```python
from build123d import *

# Parameters (mm, degrees)
SKETCH1_W           = 35
SKETCH1_H           = 35
BOSS_EXTRUDE1_DEPTH = 1
SKETCH3_R           = 11.5
SKETCH3_R_2         = 10.25
BOSS_EXTRUDE3_DEPTH = 10
FILLET1_R           = 5


with BuildPart() as part:
    # Sketch1 → Boss-Extrude1 (new body)
    with BuildSketch(Plane(origin=(0, 0, 0), x_dir=(1, 0, 0), z_dir=(0, 1, 0))):
        with Locations((17.5, 17.5)):
            Rectangle(SKETCH1_W, SKETCH1_H)
    extrude(amount=BOSS_EXTRUDE1_DEPTH)

    # Sketch3 → Boss-Extrude3 (add)
    with BuildSketch(Plane.XZ):
        with Locations(Location((17.5, -17.5, 0), (0, 0, 270))):
            Circle(SKETCH3_R)
        with Locations(Location((17.5, -17.5, 0), (0, 0, 270))):
            Circle(SKETCH3_R_2, mode=Mode.SUBTRACT)
    extrude(amount=BOSS_EXTRUDE3_DEPTH)

    # Fillet1
    # the kernel refuses this fillet: 5 mm, written as the material it takes off along each edge
    with BuildSketch(Plane(origin=(17.5, -10, -17.5), x_dir=(0, 0, -1), z_dir=(-1, 0, 0))) as fillet1_piece_1:
        with BuildLine():
            CenterArc((6.5, -3.307189139), FILLET1_R, 0, 41.409622109)
            Line((10.25, 0), (10.325, 0.066143783))
            ThreePointArc((10.325, 0.066143783), (10.875, 0.1), (11.5, 0.1))
            Line((11.5, 0.1), (11.6, 0))
            Line((11.6, 0), (11.6, -3.307189139))
            Line((11.6, -3.307189139), (11.5, -3.307189139))
        make_face()
    revolve(axis=Axis((17.5, -10, -17.5), (0, -1, 0)), mode=Mode.SUBTRACT)


solid = part.part
```
Geometry check sheet. Reference: the model listing, model coordinates, mm. A direction names the side the tool comes from. Give positions to 0.01 mm unless a question says otherwise; leave off trailing zeros. Order: outer loops, then holes, each group sorted by start corner. A loop starts at its lowest first (then second) coordinate and runs counter-clockwise, first axis right, second up. Notation, with made-up numbers: (10.25, -25) - (69.25, -25) arc R36 cw to (69.25, 13) - close; hole circle Ø9 at (-29, -33.75). An arc over 180 degrees is marked (long way). Answer in a Markdown table with one row per item. Add a question column.
Q1. Tool access check on faces 4 (the cylindrical face through (20.579, -4.93, -27.277)), 5 (the flat face through (17.3, 0.5, -35)). Record the directions out of +Z, -Z, +X, -X, +Y, -Y that give a thin tool (end or side, any length) a straight path to the whole face; none if there is none.
Q2. Cross-section at A-A, the plane x = 17.5. Enter the section's corners in (y, z).
Q3. Cross-section at B-B, the plane z = -17.5. Enter the section's corners in (x, y), then the cut area to 3 significant figures.
Q4. Mould release check, pull along X, two halves, no side actions. Record for faces 1 (the flat face through (0, 0.5, -17.3)), 2 (the flat face through (17.3, 0.5, 0)), 3 (the flat face through (17, 0, -18)): pulls with the +X half, pulls with the -X half, needs draft (parallel to the pull), parting line crosses it, or undercut.
Q5. Cross-section at C-C, the plane y = -5.5. Enter the section's corners in (x, z), then the cut area to 3 significant figures.
Q6. Gauge pin test, flat ends, axial feed: pin 1 (3 mm diameter, centred on y = -7, z = -10, fed in from -X); pin 2 (6 mm diameter, centred on x = 30.5, z = -12, fed in from -Y); pin 3 (5 mm diameter, centred on x = 16.5, y = -3.5, fed in from -Z). Record the tip position at first contact, or that the pin passes through.
Q7. Material ranges on probe 1 along X at (y, z) = (-6, -17.5); probe 2 along Y at (x, z) = (19, -19.5); probe 3 along Z at (x, y) = (13.5, -5.25), recorded low to high. Write a range as from..to.
Q8. Cross-section at D-D, the plane x = 5. Enter the section's corners in (y, z), then the cut area to 3 significant figures.
Check values:
| question | item | result |
|---|---|---|
| 1 | face 4 | -Y |
| 1 | face 5 | -Z, +X, -X, +Y, -Y |
| 2 | outline | (-10, -27.75) arc R5 ccw to (-6.69, -29) - (0, -29) - (0, -35) - (1, -35) - (1, 0) - (0, 0) - (0, -6) - (-6.69, -6) arc R5 ccw to (-10, -7.25) - (0, -7.25) - (0, -27.75) - close |
| 3 | outline | (0, 0) - (6, 0) - (6, -6.69) arc R5 ccw to (7.25, -10) - (7.25, 0) - (27.75, 0) - (27.75, -10) arc R5 ccw to (29, -6.69) - (29, 0) - (35, 0) - (35, 1) - (0, 1) - close |
| 3 | area | 57.4 mm^2 |
| 4 | face 1 | pulls with the -X half |
| 4 | face 2 | needs draft |
| 4 | face 3 | undercut |
| 5 | outline | circle Ø23 at (17.5, -17.5); hole circle Ø20.5 at (17.5, -17.5) |
| 5 | area | 85.4 mm^2 |
| 6 | pin 1 | stops at x = 7.7 |
| 6 | pin 2 | stops at y = -8.62 |
| 6 | pin 3 | stops at z = -29 |
| 7 | probe 1 | x = 6..7.25, 27.75..29 |
| 7 | probe 2 | y = 0..1 |
| 7 | probe 3 | z = -28.28..-26.94, -8.06..-6.72 |
| 8 | outline | (0, -35) - (1, -35) - (1, 0) - (0, 0) - close |
| 8 | area | 35.0 mm^2 |
